Verification items for the finished model (mm, model axes). A direction names the side the tool comes from. Give positions to 0.01 mm unless a question says otherwise; leave off trailing zeros. Write each loop counter-clockwise with the first axis right and the second up, starting at its lowest first coordinate (ties: lowest second). Pieces come first, ordered by that corner, then holes. Notation, with made-up numbers: (53.25, -16.75) - (68.25, -16.75) arc R19 cw to (68.25, 19.25) - close; hole circle Ø7 at (-11, 88.5). An arc over 180 degrees is marked (long way). Answer as a JSON object with one key per item and string values. Group by question number.
Item 1: Sectioned sample at D-D, the plane z = 49. Count the separate pieces of the cut face and the enclosed holes in it, and give its area (3 significant figures).
Item 2: Scan lines: line 1 along X through (y, z) = (14.5, 51.75); line 2 along Y through (x, z) = (30, 51.5); line 3 along X through (y, z) = (29, 53). Record each from-to range of solid material in increasing order. Write a range as [from, to].
Item 3: Sectioned sample at B-B, the plane x = 39. Record the boundary of the cut face in (y, z).
Item 4: Tool access check on faces 1 (the face through (8.353, 29, 52)), 2 (the face through (31.295, 6.244, 52.503)), 3 (the face through (-40.07, 0.99, 54.66)). Record the directions out of +Z, -Z, +X, -X, +Y, -Y that give a thin tool (end or side, any length) a straight path to the whole face; none if there is none.
Item 5: Sectioned sample at C-C, the plane y = 16.5. Record the boundary of the cut face in (x, z), and give its area (3 significant figures).
Item 6: Sectioned sample at A-A, the plane y = 28. Record the boundary of the cut face in (x, z), and give its area (3 significant figures).
Item 7: Draft check along X on faces 4 (the face through (4, 18, 47.968)), 5 (the face through (31.48, 4.42, 52.5)), 6 (the face through (56.561, 19, 57)), 7 (the face through (48.764, 32.262, 53.264)). Enter one of: +X half, -X half, draft (parallel to the pull), parting line (faces both ways), or undercut.
Item 8: Go/stop test with flat-tipped pins: pin 1 (2 mm diameter, centred on x = 30.5, y = 6.5, fed in from +Z); pin 2 (3 mm diameter, centred on x = -40.45, z = 52.95, fed in from +Y); pin 3 (3 mm diameter, centred on x = 50.5, y = 4.5, fed in from +Z). Record where each tip stops, or that it passes through.
Autodesk Inventor part; units mm, degrees
ref_plane "YZ Plane" through (0, 0, 0) normal (1, 0, 0) x (0, 1, 0)
ref_plane "XZ Plane" through (0, 0, 0) normal (0, 1, 0) x (-1, 0, 0)
ref_plane "XY Plane" through (0, 0, 0) normal (0, 0, 1) x (1, 0, 0)
sketch "Esboço1" plane through (0, 0, 0) normal (0, 1, 0) x (-1, 0, 0)
  line L0 (-56.5608, 57.9684) -> (47.4498, 57.9684)
  line L1 (47.4498, 57.9684) -> (47.4498, 47.9684)
  line L2 (-56.5608, 47.9684) -> (-56.5608, 57.9684)
  circle A0 centre (-49.5502, 52.951) radius 1.75
  circle A1 centre (40.4498, 52.951) radius 1.75
  circle A2 centre (-4.4961, 52.9684) radius 1.75
  line L3 (37.4498, 47.9684) -> (-46.5502, 47.9684)
  line L4 (43.9498, 47.9684) -> (37.2226, 47.9684)
  line L5 (37.4498, 47.9684) -> (-46.5502, 47.9684)
  line L6 (-53.0502, 47.9684) -> (-46.323, 47.9684)
  line L7 (47.4498, 47.9684) -> (-56.5608, 47.9684)
  line L8 (-53.0502, 47.9684) -> (-53.0502, 57.9684) construction
  line L9 (47.4498, 55.4684) -> (-56.5608, 55.4684)
  line L10 (-53.0502, 47.9684) -> (-53.0502, 57.9684)
  line L11 (43.9498, 47.9684) -> (43.9498, 57.9684)
  point P0 (43.9498, 55.4684)
  point P1 (-53.0502, 55.4684)
  dimension "d4" = 3.5
  dimension "d5" = 5
  dimension "d16" = 2.5
  dimension "d17" = 10
  dimension "d77" = 3.5106
  dimension "d78" = 3.5
extrude "Extrusão1" add sketch "Esboço1" along normal blind 38.5 contours L0 L10 L9 L2 | L0 L11 L9 L10 | L0 L1 L9 L11
extrude "Extrusão2" add sketch "Esboço1" along normal blind 2.5 contours L9 L11 L4 L3 L6 L10
sketch "Esboço2" plane through (-47.4498, 0, 57.9684) normal (0, 0, 1) x (1, 0, 0)
  line L0 (3.5, 36.5) -> (100.5106, 36.5)
  line L1 (100.5106, 36.5) -> (100.5106, 1.5)
  line L2 (100.5106, 1.5) -> (3.5, 1.5)
  line L3 (3.5, 1.5) -> (3.5, 36.5)
  line L4 (0, 0) -> (0, 38.5)
  line L5 (0, 38.5) -> (104.0106, 38.5)
  line L6 (0, 0) -> (104.0106, 0)
  line L7 (104.0106, 0) -> (104.0106, 38.5)
  circle A0 centre (6, 34) radius 1.75
  circle A1 centre (6, 34) radius 2.5
  circle A2 centre (6, 4) radius 1.75
  circle A3 centre (6, 4) radius 2.5
  circle A4 centre (98.0106, 34) radius 2.5
  circle A5 centre (98.0106, 34) radius 1.75
  circle A6 centre (98.0106, 4) radius 2.5
  circle A7 centre (98.0106, 4) radius 1.75
  line L8 (78.8028, 29.8071) -> (78.8028, 7.4296)
  line L9 (21.5, 17) -> (31.5, 17)
  line L10 (31.5, 17) -> (31.5, 7)
  line L11 (31.5, 7) -> (21.5, 7)
  line L12 (21.5, 7) -> (21.5, 17)
  line L13 (35.5, 23.5) -> (45.5, 23.5)
  line L14 (45.5, 23.5) -> (45.5, 13.5)
  line L15 (45.5, 13.5) -> (35.5, 13.5)
  line L16 (35.5, 13.5) -> (35.5, 23.5)
  line L17 (21.5, 31.5) -> (31.5, 31.5)
  line L18 (31.5, 31.5) -> (31.5, 21.5)
  line L19 (31.5, 21.5) -> (21.5, 21.5)
  line L20 (21.5, 21.5) -> (21.5, 31.5)
  line L21 (7.5, 23.5) -> (17.5, 23.5)
  line L22 (17.5, 23.5) -> (17.5, 13.5)
  line L23 (17.5, 13.5) -> (7.5, 13.5)
  line L24 (7.5, 13.5) -> (7.5, 23.5)
  line L25 (83.324, 31) -> (93.324, 31)
  line L26 (93.324, 31) -> (93.324, 11)
  line L27 (93.324, 11) -> (83.324, 11)
  line L28 (83.324, 11) -> (83.324, 31)
  circle A8 centre (26.5, 26.5) radius 3.5
  circle A9 centre (40.5, 18.5) radius 3.5
  circle A10 centre (26.5, 11.5) radius 3.5
  circle A11 centre (12.5, 18.5) radius 3.5
  line L29 (8.2913, 35) -> (95.7193, 35)
  line L30 (5, 6.2913) -> (5, 31.7087)
  line L31 (95.7193, 3) -> (8.2913, 3)
  line L32 (99.0106, 31.7087) -> (99.0106, 6.2913)
  circle A12 centre (52.0528, 31.3683) radius 1.25
  circle A13 centre (77.5528, 5.8683) radius 1.25
  circle A14 centre (77.5528, 31.3683) radius 1.25
  circle A15 centre (52.0528, 5.8683) radius 1.25
  circle A16 centre (52.0528, 5.8683) radius 2
  circle A17 centre (52.0528, 31.3683) radius 2
  circle A18 centre (77.5528, 31.3683) radius 2
  circle A19 centre (77.5528, 5.8683) radius 2
  line L33 (55.8028, 32.6183) -> (73.8028, 32.6183)
  line L34 (73.8028, 32.6183) -> (73.8028, 25.6183)
  line L35 (73.8028, 25.6183) -> (55.8028, 25.6183)
  line L36 (55.8028, 25.6183) -> (55.8028, 32.6183)
  line L37 (50.8028, 7.4296) -> (50.8028, 29.8071)
  line L38 (50.8028, 31.3683) -> (50.8028, 31.5)
  line L39 (53.6141, 32.6183) -> (75.9916, 32.6183)
  line L40 (78.8028, 4.6183) -> (77.5528, 4.6183)
  line L41 (75.9916, 4.6183) -> (53.6141, 4.6183)
  line L42 (52.0528, 4.6183) -> (50.8028, 4.6183)
  point P0 (47.4498, 0)
  point P1 (26.5, 17)
  point P2 (64.8028, 25.6183)
  point P3 (64.8028, 32.6183)
  dimension "d81" = 2.5
  dimension "d82" = 2.5
  dimension "d84" = 2.5
  dimension "d22" = 3.5
  dimension "d23" = 2
  dimension "d25" = 3.5
  dimension "d26" = 3.5
  dimension "d27" = 5
  dimension "d28" = 3.5
  dimension "d29" = 5
  dimension "d30" = 5
  dimension "d31" = 3.5
  dimension "d32" = 5
  dimension "d33" = 3.5
  dimension "d34" = 104.0106
  dimension "d35" = 38.5
  dimension "d36" = 28
  dimension "d38" = 10
  dimension "d39" = 10
  dimension "d40" = 10
  dimension "d41" = 10
  dimension "d42" = 10
  dimension "d43" = 10
  dimension "d44" = 10
  dimension "d45" = 10
  dimension "d46" = 10
  dimension "d47" = 20
  dimension "d49" = 4
  dimension "d50" = 4
  dimension "d51" = 4
  dimension "d52" = 4
  dimension "d57" = 5.5
  dimension "d58" = 7
  dimension "d59" = 7
  dimension "d60" = 7
  dimension "d61" = 7
  dimension "d65" = 1.5
  dimension "d72" = 4.5
  dimension "d83" = 2.5
  dimension "d85" = 4
  dimension "d86" = 4
  dimension "d87" = 4
  dimension "d88" = 4
  dimension "d90" = 5
  dimension "d91" = 7
extrude "Extrusão3" add sketch "Esboço2" against normal blind 10 contours L0 A1 L3 | L0 A4 L29 A1 | A1 | A1 L30 A3 L3 | L0 L1 A4 | A4 | L29 A4 L32 A6 L31 A3 L30 A1 | A3 L2 L3 | A3 | L1 A6 L32 A4 | A3 L31 A6 L2 | A6 | L1 L2 A6 | A0 | A2 | A5 | A7 | L8 A19 L41 A16 L37 A17 L39 L36 L35 L34 A18 | A18 | A19 | L34 L35 L36 L33 | A16 | A17 | L9 L10 L11 L12 | L13 L14 L15 L16 | L17 L18 L19 L20 | L21 L22 L23 L24 | L25 L26 L27 L28 | A8 | A9 | A10 | A11 | A12 | A13 | A14 | A15
extrude "Extrusão4" cut sketch "Esboço2" against normal blind 8 contours L29 A4 L32 A6 L31 A3 L30 A1 | L8 A19 L41 A16 L37 A17 L39 L36 L35 L34 A18 | A18 | A19 | L34 L35 L36 L33 | A16 | A17 | L9 L10 L11 L12 | L13 L14 L15 L16 | L17 L18 L19 L20 | L21 L22 L23 L24 | L25 L26 L27 L28 | A8 | A9 | A10 | A11 | A12 | A13 | A14 | A15
extrude "Extrusão5" cut sketch "Esboço2" against normal blind 1.5 contours L0 A1 L3 | L0 A4 L29 A1 | A1 | A1 L30 A3 L3 | L0 L1 A4 | A4 | A3 L2 L3 | A3 | L1 A6 L32 A4 | A3 L31 A6 L2 | A6 | L1 L2 A6 | A0 | A2 | A5 | A7
extrude "Extrusão6" cut sketch "Esboço2" against normal blind 8 contours A0 | A2 | A5 | A7
extrude "Extrusão7" cut sketch "Esboço2" against normal through all contours L25 L26 L27 L28
extrude "Extrusão8" cut sketch "Esboço1" along normal blind 2 contours A0 | A1 | A2
extrude "Extrusão9" add sketch "Esboço2" against normal blind 8.5 contours L8 A19 L41 A16 L37 A17 L39 L36 L35 L34 A18 | A18 | A19 | A16 | A17
extrude "Extrusão10" cut sketch "Esboço2" against normal blind 3 contours L8 A19 L41 A16 L37 A17 L39 L36 L35 L34 A18 | A18 | A19 | A16 | A17 | A13 | A14 | A15
extrude "Extrusão11" cut sketch "Esboço2" against normal through all contours L34 L35 L36 L33
properties part number "suporte_lcd_botoes"
Geometry check:
{
 "1": {"separate pieces": "1", "enclosed holes": "2", "area": "3,210 mm^2"},
 "2": {"line 1": "[-43.95, -42.45], [3.35, 31.35], [51.56, 53.06]", "line 2": "[0, 3], [3.87, 4.62], [7.11, 30.12], [32.61, 33.37], [35, 36.5]", "line 3": "[-43.95, -42.45], [3.35, 8.35], [26.35, 31.35], [51.56, 53.06]"},
 "3": {"outline": "(0, 47.97) - (11, 47.97) - (11, 49.97) - (3, 49.97) - (3, 56.47) - (1.5, 56.47) - (1.5, 57.97) - (0, 57.97) - close; (31, 47.97) - (36.5, 47.97) - (36.5, 55.47) - (38.5, 55.47) - (38.5, 57.97) - (36.5, 57.97) - (36.5, 56.47) - (35, 56.47) - (35, 49.97) - (31, 49.97) - close"},
 "4": {"face 1": "+Z, -Z", "face 2": "+Z", "face 3": "-Y"},
 "5": {"outline": "(-47.45, 55.47) - (-43.95, 55.47) - (-43.95, 47.97) - (35.87, 47.97) - (35.87, 49.97) - (31.35, 49.97) - (31.35, 54.97) - (3.35, 54.97) - (3.35, 49.97) - (-42.45, 49.97) - (-42.45, 56.47) - (-43.95, 56.47) - (-43.95, 57.97) - (-47.45, 57.97) - close; (45.87, 47.97) - (53.06, 47.97) - (53.06, 55.47) - (56.56, 55.47) - (56.56, 57.97) - (53.06, 57.97) - (53.06, 56.47) - (51.56, 56.47) - (51.56, 49.97) - (45.87, 49.97) - close", "area": "351 mm^2"},
 "6": {"outline": "(-47.45, 55.47) - (-43.95, 55.47) - (-43.95, 47.97) - (8.35, 47.97) - (8.35, 54.97) - (3.35, 54.97) - (3.35, 49.97) - (-42.45, 49.97) - (-42.45, 56.47) - (-43.95, 56.47) - (-43.95, 57.97) - (-47.45, 57.97) - close; (26.35, 47.97) - (35.87, 47.97) - (35.87, 49.97) - (31.35, 49.97) - (31.35, 54.97) - (26.35, 54.97) - close; (45.87, 47.97) - (53.06, 47.97) - (53.06, 55.47) - (56.56, 55.47) - (56.56, 57.97) - (53.06, 57.97) - (53.06, 56.47) - (51.56, 56.47) - (51.56, 49.97) - (45.87, 49.97) - close", "area": "225 mm^2"},
 "7": {"face 4": "draft", "face 5": "undercut", "face 6": "+X half", "face 7": "undercut"},
 "8": {"pin 1": "z = 54.97", "pin 2": "y = 36.5", "pin 3": "z = 56.47"}
}
